CAD build for the part. Positions are in the model's coordinates, mm. A direction names the side the tool comes from. Give positions to 0.01 mm unless a question says otherwise; leave off trailing zeros. Write each loop counter-clockwise with the first axis right and the second up, starting at its lowest first coordinate (ties: lowest second). Pieces come first, ordered by that corner, then holes. Notation, with made-up numbers: (26.25, -2.5) -> (54.25, -2.5) arc R35 cw to (54.25, 35.5) -> close; hole circle Ø3 at (24, 78). An arc over 180 degrees is marked (long way). Answer as a JSON object with one key per item and string values.
```python
from build123d import *

# Parameters (mm, degrees)
FILLET2_R           = 1.5
SKETCH3_R           = 2
BOSS_EXTRUDE1_DEPTH = 3


with BuildPart() as part:
    # Sketch2 → Revolve1 (revolve)
    with BuildSketch(Plane.XY):
        Polygon((0, -30.015007431), (8, -30.015007431), (8, -23.015007431), (4.5, -23.015007431), (4.5, -22.015007431), (1.5, -20.015007431), (1.5, -18.015007431), (0, -18.015007431), align=None)
    revolve(axis=Axis((0, 46.076216781, 0), (0, -1, 0)))

    # Fillet2
    fillet2_edges = [part.edges().sort_by_distance(p)[0] for p in [
        (-8, -23.015007431, 0),
    ]]
    fillet(fillet2_edges, radius=FILLET2_R)

    # Sketch3 → Boss-Extrude1 (add)
    with BuildSketch(Plane.XZ.offset(30.015007431)):
        Circle(SKETCH3_R)
    extrude(amount=BOSS_EXTRUDE1_DEPTH)


solid = part.part
```
1) Slice it at C-C (y = -29.75). List the corners of the cut face in (x, z), then the cut area to 3 significant figures.
Model answer:
{"outline": "circle Ø16 at (0, 0)", "area": "201 mm2"}
2) 3-axis set-ups, long thin cutter, end or side, ignore diameter. For faces 1 (the flat face through (0, -18.015, 0)), 2 (the cylindrical face through (-0.59, -22.51, 4.46)), 3 (the cylindrical face through (0, -31, -2)): which of +Z, -Z, +X, -X, +Y, -Y reach the whole face in a straight line?
Model answer:
{"face 1": "+Z, -Z, +X, -X, +Y", "face 2": "+Y", "face 3": "-Y"}
3) Pin check, flat tips, straight feed: pin 1 (1 mm diameter, centred on x = 3, z = -2, fed in from +Y); pin 2 (5 mm diameter, centred on y = -28.5, z = -3, fed in from -X); pin 3 (6 mm diameter, centred on x = 6.5, y = -25, fed in from +Z); pin 4 (6 mm diameter, centred on x = 2, z = 0, fed in from +Y) (3 decimals). Stop position of each tip, or through.
Model answer:
{"pin 1": "stops at y = -21.09", "pin 2": "stops at x = -7.98", "pin 3": "stops at z = 7.19", "pin 4": "stops at y = -18.015"}
4) Slice it at D-D (y = -20.75). List the corners of the cut face in (x, z).
Model answer:
{"outline": "circle Ø5.2 at (0, 0)"}
5) Wall check: probe 1 along Y at (x, z) = (-4.75, 3.5) (3 decimals); probe 2 along Y at (x, z) = (6.5, -2.25) (3 decimals); probe 3 along X at (y, z) = (-24.75, -1). Give the ranges that are in metal, low to high.
Model answer:
{"probe 1": "y = -30.015 to -23.015", "probe 2": "y = -30.015 to -23.064", "probe 3": "x = -7.94 to 7.94"}
6) Slice it at B-B (x = 0). List the corners of the cut face in (y, z) (3 decimals), then the cut area to 3 significant figures.
Model answer:
{"outline": "(-33.015, -2) -> (-30.015, -2) -> (-30.015, -8) -> (-24.515, -8) arc R1.5 ccw to (-23.015, -6.5) -> (-23.015, -4.5) -> (-22.015, -4.5) -> (-20.015, -1.5) -> (-18.015, -1.5) -> (-18.015, 1.5) -> (-20.015, 1.5) -> (-22.015, 4.5) -> (-23.015, 4.5) -> (-23.015, 6.5) arc R1.5 ccw to (-24.515, 8) -> (-30.015, 8) -> (-30.015, 2) -> (-33.015, 2) -> close", "area": "150 mm2"}
7) Slice it at A-A (z = 0). List the corners of the cut face in (x, y) (3 decimals), then the cut area to 3 significant figures.
Model answer:
{"outline": "(-8, -30.015) -> (-2, -30.015) -> (-2, -33.015) -> (2, -33.015) -> (2, -30.015) -> (8, -30.015) -> (8, -24.515) arc R1.5 ccw to (6.5, -23.015) -> (4.5, -23.015) -> (4.5, -22.015) -> (1.5, -20.015) -> (1.5, -18.015) -> (-1.5, -18.015) -> (-1.5, -20.015) -> (-4.5, -22.015) -> (-4.5, -23.015) -> (-6.5, -23.015) arc R1.5 ccw to (-8, -24.515) -> close", "area": "150 mm2"}
